```python
from build123d import *

# Parameters (mm, degrees)
BOSS_EXTRUDE1_DEPTH = 2.3622
SKETCH2_W           = 3.175
SKETCH2_H           = 3.175
CUT_EXTRUDE1_DEPTH  = 2.54


with BuildPart() as part:
    # Sketch1 → Boss-Extrude1 (new body)
    with BuildSketch(Plane(origin=(0, 0, 0), x_dir=(1, 0, 0), z_dir=(0, 1, 0))):
        Polygon((5.7912, 6.35), (5.7912, 19.05), (2.6162, 19.05), (2.6162, 12.0142), (0, 12.0142), (0, 19.05), (-6.35, 19.05), (-6.35, 12.0142), (-22.7838, 12.0142), (-22.7838, 21.5392), (-29.1338, 21.5392), (-29.1338, 12.7), (-46.3042, 12.7), (-46.3042, 21.5392), (-52.6542, 21.5392), (-52.6542, 12.0142), (-69.088, 12.0142), (-69.088, 19.05), (-75.438, 19.05), (-75.438, 12.0142), (-78.0542, 12.0142), (-78.0542, 19.05), (-81.2292, 19.05), (-81.2292, 6.35), (-75.438, 6.35), (-75.438, 0), (0, 0), (0, 6.35), align=None)
    extrude(amount=BOSS_EXTRUDE1_DEPTH)

    # Sketch2 → Cut-Extrude1 (cut)
    with BuildSketch(Plane(origin=(0, 2.3622, 0), x_dir=(1, 0, 0), z_dir=(0, 1, 0))):
        with Locations((4.2037, 17.4625)):
            Rectangle(SKETCH2_W, SKETCH2_H)
        with Locations((-79.6417, 17.4625)):
            Rectangle(SKETCH2_W, SKETCH2_H)
    extrude(amount=-CUT_EXTRUDE1_DEPTH, mode=Mode.SUBTRACT)


solid = part.part
```
Geometry check sheet. Reference: the model listing, model coordinates, mm. A direction names the side the tool comes from. Give positions to 0.01 mm unless a question says otherwise; leave off trailing zeros. Write each loop counter-clockwise with the first axis right and the second up, starting at its lowest first coordinate (ties: lowest second). Pieces come first, ordered by that corner, then holes. Notation, with made-up numbers: (16, 61.25) -> (71, 61.25) arc R22 cw to (71, 100.25) -> close; hole circle Ø5 at (33, -4). An arc over 180 degrees is marked (long way). Use one line per item in the form item = value.
Item 1: Sectioned sample at D-D on z = -3.75. Enter the section's corners in (x, y).
Results list:
outline = (-75.44, 0) -> (0, 0) -> (0, 2.36) -> (-75.44, 2.36) -> close
Item 2: Sectioned sample at A-A on z = -17.75. Enter the section's corners in (x, y), plus the area to 3 significant figures.
Results list:
outline = (-75.44, 0) -> (-69.09, 0) -> (-69.09, 2.36) -> (-75.44, 2.36) -> close; (-52.65, 0) -> (-46.3, 0) -> (-46.3, 2.36) -> (-52.65, 2.36) -> close; (-29.13, 0) -> (-22.78, 0) -> (-22.78, 2.36) -> (-29.13, 2.36) -> close; (-6.35, 0) -> (0, 0) -> (0, 2.36) -> (-6.35, 2.36) -> close
area = 60.0 mm2
Item 3: Depth check by flat-ended pin: pin 1 Ø1.2 at (x, y) = (-73.5, 1) entering from -Z; pin 2 Ø1.2 at (x, y) = (-33.5, 1) entering from -Z; pin 3 Ø1 at (y, z) = (2, -3) entering from +X; pin 4 Ø5 at (x, z) = (-34, -14.5) entering from -Y. Enter the tip coordinate at first touch or a pass-through.
Results list:
pin_1 = -19.05
pin_2 = -12.7
pin_3 = 0
pin_4 = 0
Item 4: Access from +Z, -Z, +X, -X, +Y, -Y to the whole of each face (thin tool, end or side, straight path). Record for faces 1 (the flat face through (1, 1, -12.014)), 2 (the flat face through (-80, 1, -15.875)), 3 (the flat face through (-78, 1, -6.35)).
Results list:
face_1 = -Z, +Y, -Y
face_2 = -Z, -X, +Y, -Y
face_3 = +Z, -X, +Y, -Y
Item 5: Scan lines: line 1 (X direction, y = 1.4, z = -17.25); line 2 (X direction, y = 1.8, z = -14); line 3 (X direction, y = 0.45, z = -19.5). Record each from-to range of solid material in increasing order.
Results list:
line_1 = -75.44 to -69.09, -52.65 to -46.3, -29.13 to -22.78, -6.35 to 0
line_2 = -81.23 to -78.05, -75.44 to -69.09, -52.65 to -46.3, -29.13 to -22.78, -6.35 to 0, 2.62 to 5.79
line_3 = -52.65 to -46.3, -29.13 to -22.78
Item 6: Mould release check, pull along X, two halves, no side actions. Record for faces 4 (the flat face through (0, 1, -3)), 5 (the flat face through (-75.438, 1, -16)), 6 (the flat face through (4, 1, -15.875)): released by +X, released by -X, zero draft, split by the parting line, or undercut.
Results list:
face_4 = released by +X
face_5 = undercut
face_6 = zero draft
Item 7: Sectioned sample at C-C on x = -4.5. Enter the section's corners in (y, z), plus the area to 3 significant figures.
Results list:
outline = (0, -19.05) -> (2.36, -19.05) -> (2.36, 0) -> (0, 0) -> close
area = 45.0 mm2
Item 8: Sectioned sample at B-B on y = 0.4. Enter the section's corners in (x, z) (3 decimals).
Results list:
outline = (-81.229, -15.875) -> (-78.054, -15.875) -> (-78.054, -12.014) -> (-75.438, -12.014) -> (-75.438, -19.05) -> (-69.088, -19.05) -> (-69.088, -12.014) -> (-52.654, -12.014) -> (-52.654, -21.539) -> (-46.304, -21.539) -> (-46.304, -12.7) -> (-29.134, -12.7) -> (-29.134, -21.539) -> (-22.784, -21.539) -> (-22.784, -12.014) -> (-6.35, -12.014) -> (-6.35, -19.05) -> (0, -19.05) -> (0, -12.014) -> (2.616, -12.014) -> (2.616, -15.875) -> (5.791, -15.875) -> (5.791, -6.35) -> (0, -6.35) -> (0, 0) -> (-75.438, 0) -> (-75.438, -6.35) -> (-81.229, -6.35) -> close
